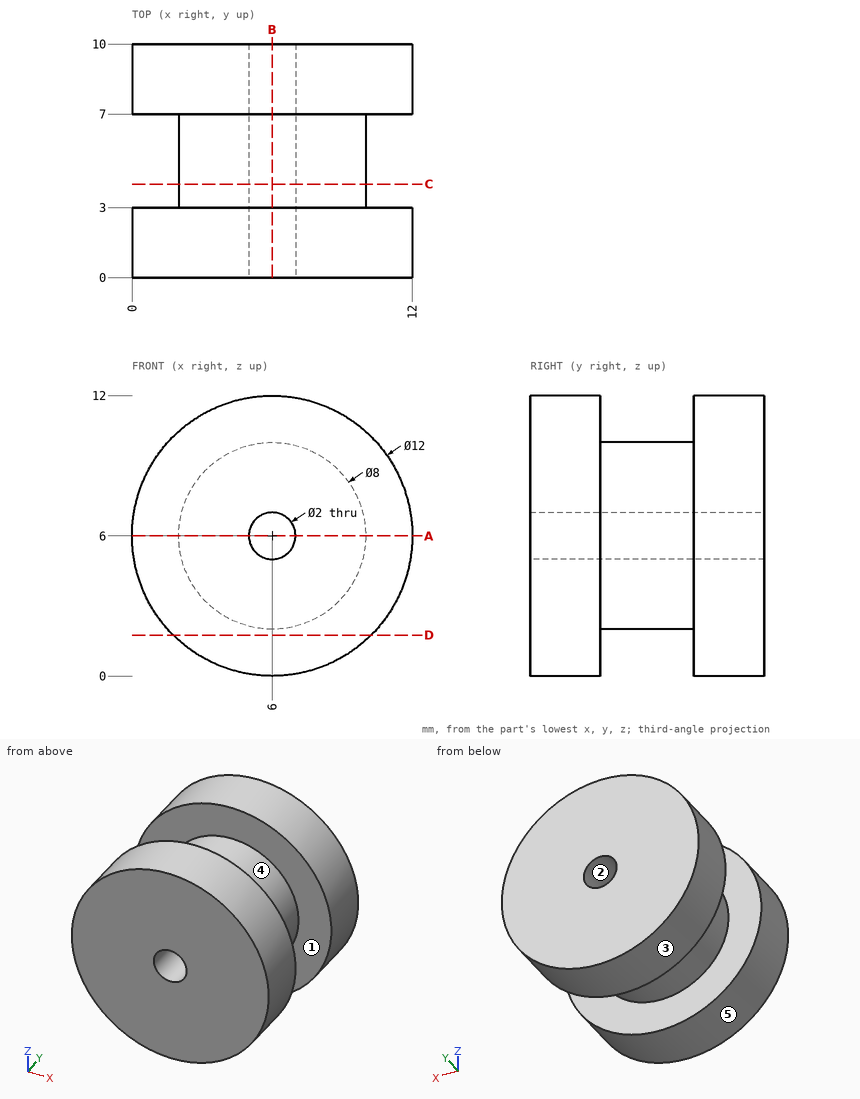
Input: dimensioned drawing with shaded views. Units: mm. Origin: part minimum x, y, z. A direction names the side the tool comes from. Coordinates: 2 decimals unless noted, no trailing zeros. Loops run counter-clockwise (first coordinate to the right, second up) from the corner with the lowest first, then second, coordinate; pieces in that order, holes last. Notation, with made-up numbers: M -35,20.25 L 0,20.25 A30 ccw 0,47.25 Z; hole C 47,53 d7. An arc over 180 degrees is marked long. Put each result on its own line as item: value.
(1) Cut plane D-D on z = 1.75. Return the cut outline in (x, y).
Answer sheet:
outline: M 1.76,0 L 10.24,0 L 10.24,3 L 1.76,3 Z; M 1.76,7 L 10.24,7 L 10.24,10 L 1.76,10 Z
(2) Access query for the marked faces 4 and 5. Directions: +Z, -Z, +X, -X, +Y, -Y. A direction counts if a zero-diameter tool reaches every point of the face in a straight line with its end or side. Return the directions, or none.
Answer sheet:
face 4: none
face 5: +Y, -Y
(3) Cut plane A-A on z = 6. Return the cut outline in (x, y).
Answer sheet:
outline: M 0,0 L 5,0 L 5,10 L 0,10 L 0,7 L 2,7 L 2,3 L 0,3 Z; M 7,0 L 12,0 L 12,3 L 10,3 L 10,7 L 12,7 L 12,10 L 7,10 Z
(4) Cut plane C-C on y = 4. Return the cut outline in (x, z), then the cut area to 3 significant figures.
Answer sheet:
outline: C 6,6 d8; hole C 6,6 d2
area: 47.1 mm^2
(5) Draft query along Z for the marked faces 1, 2 and 3. Return one class per face: pulls with the +Z half, pulls with the -Z half, needs draft (parallel to the pull), parting line crosses it, or undercut.
Answer sheet:
face 1: needs draft
face 2: undercut
face 3: parting line crosses it
(6) First-contact query: pin 1 (3 mm diameter, centred on x = 8, y = 4, fed in from -Z); pin 2 (1 mm diameter, centred on x = 2, y = 4, fed in from -Z). Flat tips, straight axial feed; report the tip coordinate or a pass-through.
Answer sheet:
pin 1: stops at z = 0.07
pin 2: stops at z = 4.06
(7) Cut plane B-B on x = 6. Return the cut outline in (y, z), then the cut area to 3 significant figures.
Answer sheet:
outline: M 0,0 L 3,0 L 3,2 L 7,2 L 7,0 L 10,0 L 10,5 L 0,5 Z; M 0,7 L 10,7 L 10,12 L 7,12 L 7,10 L 3,10 L 3,12 L 0,12 Z
area: 84.0 mm^2
(8) Material intervals for probe 1 along Y at (x, z) = (6.25, 1.25); probe 2 along X at (y, z) = (4.5, 6), sorted ascending.
Answer sheet:
probe 1: y = 0 to 3, 7 to 10
probe 2: x = 2 to 5, 7 to 10
